```python
from build123d import *

# Parameters (mm, degrees)
SKETCH1_R           = 1.6
BOSS_EXTRUDE1_DEPTH = 4
FILLET2_R           = 3


with BuildPart() as part:
    # Sketch1 → Boss-Extrude1 (new body)
    # profile 1 of 3: a face of its own
    with BuildSketch(Plane.XY):
        Polygon((-2.008891974, 36.379591132), (7.987954355, 36.630715556), (8.741327627, 6.640176569), (-1.255518702, 6.389052145), align=None)
        with Locations((3.617342251, 11.513037521)):
            Circle(SKETCH1_R, mode=Mode.SUBTRACT)
        with Locations((3.115093403, 31.506730179)):
            Circle(SKETCH1_R, mode=Mode.SUBTRACT)
    # profile 2 of 3: a face of its own
    with BuildSketch(Plane.XY):
        Polygon((28.735020285, 7.142425417), (7.987954355, 36.630715556), (8.741327627, 6.640176569), align=None)
    # profile 3 of 3: a face of its own
    with BuildSketch(Plane.XY):
        Polygon((28.986144709, -2.854420912), (28.735020285, 7.142425417), (8.741327627, 6.640176569), (-1.255518702, 6.389052145), (-1.004394278, -3.607794184), align=None)
        with Locations((3.868466675, 1.516191192)):
            Circle(SKETCH1_R, mode=Mode.SUBTRACT)
        with Locations((23.862159332, 2.018440041)):
            Circle(SKETCH1_R, mode=Mode.SUBTRACT)
    extrude(amount=BOSS_EXTRUDE1_DEPTH)

    # Fillet2
    fillet2_edges = [part.edges().sort_by_distance(p)[0] for p in [
        (28.986144709, -2.854420912, 2),
        (-1.004394278, -3.607794184, 2),
        (-2.008891974, 36.379591132, 2),
        (7.987954355, 36.630715556, 2),
        (28.735020285, 7.142425417, 2),
    ]]
    fillet(fillet2_edges, radius=FILLET2_R)


solid = part.part
```
Source: CAD feature listing. Evaluate the final solid. Frame: model axes, mm. Give positions to 0.01 mm unless a question says otherwise; leave off trailing zeros. Write each loop counter-clockwise with the first axis right and the second up, starting at its lowest first coordinate (ties: lowest second). Pieces come first, ordered by that corner, then holes.
1. Material intervals for line 1 along X through (y, z) = (1.5, 3.6); line 2 along X through (y, z) = (2, 1.7); line 3 along Y through (x, z) = (23, 3.35), sorted ascending.
2. Section query D-D (y = 24). Return the cut outline in (x, z).
3. Pull-direction query (Y, two-part tool) for faces 1 (the face through (28.61, 7.09, 2.03)), 2 (the face through (22.264, 2.089, 1.972)), 3 (the face through (10, 12, 0)); classes: +Y half, -Y half, draft (parallel to the pull), parting line (faces both ways), or undercut.
4. Section query A-A (x = 24). Return the cut outline in (y, z), then the cut area to 3 significant figures.
5. Section query B-B (z = 0.75). Return the cut outline in (x, y), then the cut area to 3 significant figures.
6. First-contact query: pin 1 (1.5 mm diameter, centred on y = 32, z = 2, fed in from -X); pin 2 (1 mm diameter, centred on x = 16, z = 1, fed in from -Y); pin 3 (2.5 mm diameter, centred on x = 3.62, y = 11.51, fed in from -Z). Flat tips, straight axial feed; report the tip coordinate or a pass-through.
7. Section query C-C (y = 31). Return the cut outline in (x, z), then the cut area to 3 significant figures.
Output values:
1. line 1: x = -1.13 to 2.27, 5.47 to 22.35, 25.38 to 28.88
1. line 2: x = -1.15 to 2.34, 5.39 to 22.26, 25.46 to 28.86
1. line 3: y = -3 to 0.67, 3.37 to 15.29
2. outline: (-1.7, 0) - (16.87, 0) - (16.87, 4) - (-1.7, 4) - close
3. face 1: +Y half
3. face 2: undercut
3. face 3: draft
4. outline: (-2.98, 0) - (0.42, 0) - (0.42, 4) - (-2.98, 4) - close; (3.61, 0) - (13.87, 0) - (13.87, 4) - (3.61, 4) - close
4. area: 54.7 mm2
5. outline: (-1.93, 33.38) - (-1.08, -0.61) arc R3 ccw to (1.99, -3.53) - (25.99, -2.93) arc R3 ccw to (28.91, 0.14) - (28.76, 6.23) arc R3 ccw to (28.21, 7.89) - (8.91, 35.32) arc R3 ccw to (6.38, 36.59) - (0.99, 36.45) arc R3 ccw to start; hole circle Ø3.2 at (3.12, 31.51); hole circle Ø3.2 at (3.62, 11.51); hole circle Ø3.2 at (3.87, 1.52); hole circle Ø3.2 at (23.86, 2.02)
5. area: 862 mm2
6. pin 1: stops at x = -1.92
6. pin 2: stops at y = -3.19
6. pin 3: passes through
7. outline: (-1.87, 0) - (1.6, 0) - (1.6, 4) - (-1.87, 4) - close; (4.63, 0) - (11.95, 0) - (11.95, 4) - (4.63, 4) - close
7. area: 43.2 mm2
